```python
from build123d import *

# Parameters (mm, degrees)
CROQUIS1_R              = 4.5
SALIENTE_EXTRUIR1_DEPTH = 2
CROQUIS2_R              = 2
SALIENTE_EXTRUIR2_DEPTH = 13
REDONDEO1_R             = 2
CROQUIS3_R              = 3
SALIENTE_EXTRUIR3_DEPTH = 1
REDONDEO2_R             = 0.5


with BuildPart() as part:
    # Croquis1 → Saliente-Extruir1 (new body)
    with BuildSketch(Plane(origin=(0, 0, 0), x_dir=(1, 0, 0), z_dir=(0, 1, 0))):
        with Locations(Location((0, 0, 0), (0, 0, 270))):
            Circle(CROQUIS1_R)
    extrude(amount=SALIENTE_EXTRUIR1_DEPTH)

    # Croquis2 → Saliente-Extruir2 (add)
    with BuildSketch(Plane.XZ):
        with Locations(Location((0, 0, 0), (0, 0, 90))):
            Circle(CROQUIS2_R)
    extrude(amount=SALIENTE_EXTRUIR2_DEPTH)

    # Redondeo1
    redondeo1_edges = [part.edges().sort_by_distance(p)[0] for p in [
        (0, 2, -4.5),
    ]]
    fillet(redondeo1_edges, radius=REDONDEO1_R - 0.0001)  # a hair under: the kernel refuses the full size

    # Croquis3 → Saliente-Extruir3 (add)
    with BuildSketch(Plane(origin=(0, -13, 0), x_dir=(-1, 0, 0), z_dir=(0, -1, 0))):
        with Locations(Location((0, 0, 0), (0, 0, 90))):
            Circle(CROQUIS3_R)
    extrude(amount=SALIENTE_EXTRUIR3_DEPTH)

    # Redondeo2
    redondeo2_edges = [part.edges().sort_by_distance(p)[0] for p in [
        (0, -14, 3),
    ]]
    fillet(redondeo2_edges, radius=REDONDEO2_R)


solid = part.part
```
Geometry: final body of the model. Coordinates: model frame, mm. Round coordinates to 2 decimals unless told otherwise and drop trailing zeros. Order: outer loops, then holes, each group sorted by start corner. A loop starts at its lowest first (then second) coordinate and runs counter-clockwise, first axis right, second up. Notation, with made-up numbers: (36.5, -31.5) -> (67.5, -31.5) arc R22 cw to (67.5, -16.5) -> close; hole circle Ø8 at (-25.5, 89.25). An arc over 180 degrees is marked (long way). Use one line per item in the form item = value. Start each with the question number.
1. Line query: probe 1 along Y at (x, z) = (-1, -2.25); probe 2 along Y at (x, z) = (-2, 2); probe 3 along X at (y, z) = (-0.5, 0). Output: solid intervals per line, ascending.
2. Pin query (flat end, axial travel): pin 1 Ø5 at (x, z) = (3.5, 1.5) entering from +Y; pin 2 Ø2 at (x, y) = (3.5, -6.5) entering from -Z. Return the tip coordinate at first contact, or that it passes through.
3. Cut plane C-C (y = -8.75). Return the cut outline in (x, z).
4. Draft query along Y for faces 1 (the face through (0.9, -13.25, -2.86)), 2 (the face through (0, 2, 0)), 3 (the face through (2, -6, 0)), 4 (the face through (0, -14, 0)). Return one class per face: pulls with the +Y half, pulls with the -Y half, needs draft (parallel to the pull), parting line crosses it, or undercut.
Solution:
q1.probe_1 = -14 to -13, 0 to 2
q1.probe_2 = -13.88 to -13, 0 to 1.97
q1.probe_3 = -2 to 2
q2.pin_1 = 2
q2.pin_2 = through
q3.outline = circle Ø4 at (0, 0)
q4.face_1 = needs draft
q4.face_2 = pulls with the +Y half
q4.face_3 = undercut
q4.face_4 = pulls with the -Y half
